```python
from build123d import *

# Parameters (mm, degrees)
F0_W     = 1143
F0_H     = 635
F1_DEPTH = 25.4
F2_W     = 76.2
F2_H     = 76.2
F3_DEPTH = 889


with BuildPart() as f1:
    # F0 (on Top) → F1 (new body, symmetric)
    with BuildSketch(Plane.XY):
        Rectangle(F0_W, F0_H)
    extrude(amount=F1_DEPTH, both=True)

    # F2 (on face) → F3 (join)
    with BuildSketch(Plane.XY.offset(25.4)):
        with Locations((-533.4, 279.4)):
            Rectangle(F2_W, F2_H)
        with Locations((-533.4, -279.4)):
            Rectangle(F2_W, F2_H)
        with Locations((533.4, 279.4)):
            Rectangle(F2_W, F2_H)
        with Locations((533.4, -279.4)):
            Rectangle(F2_W, F2_H)
    extrude(amount=F3_DEPTH)


solid = f1.part
```
The model under review builds one solid part; all positions refer to its coordinate system, in mm. A direction names the side the tool comes from. Round coordinates to 2 decimals unless told otherwise and drop trailing zeros. Write each loop counter-clockwise with the first axis right and the second up, starting at its lowest first coordinate (ties: lowest second). Pieces come first, ordered by that corner, then holes. Notation, with made-up numbers: (53.5, -13.5) - (90.5, -13.5) arc R30 cw to (90.5, 9.5) - close; hole circle Ø3 at (-9.5, 76). An arc over 180 degrees is marked (long way). Answer as CSV lines item,"result". Start each with the question number.
(1) To check wall thickness, follow line 1 (Y direction, x = 512, z = 719); line 2 (Z direction, x = -198, y = -113.5). State the ranges of each line that lie inside material, in increasing order.
(2) For faces 1 (the flat face through (495.3, -280, 464)), 2 (the flat face through (533, -241.3, 464)), 3 (the flat face through (571.5, -260, 377)), list the 3-axis set-ups (+Z, -Z, +X, -X, +Y, -Y) from which the entire face can be reached by the end or side of a thin tool; tool diameter is ignored.
(3) Draft analysis for pull direction X (two halves, no side actions). For faces 4 (the flat face through (-571.5, -260, 338)), 5 (the flat face through (533, 241.3, 464)), 6 (the flat face through (-8, 4, 25.4)), state which applies: pulls with the +X half, pulls with the -X half, needs draft (parallel to the pull), parting line crosses it, or undercut.
(4) We need section A-A on z = 473.5. State the section outline as (x, y) points.
(5) We need section C-C on x = 185. State the section outline as (y, z) points, plus the area to 3 significant figures.
(6) We need section B-B on y = -213.5. State the section outline as (x, z) points, plus the area to 3 significant figures.
Worked answers:
1,line 1,"-317.5 to -241.3, 241.3 to 317.5"
1,line 2,"-25.4 to 25.4"
2,face 1,"+Z, +Y, -Y"
2,face 2,"+Z, +X, -X"
2,face 3,"+Z, -Z, +X, +Y, -Y"
3,face 4,"pulls with the -X half"
3,face 5,"needs draft"
3,face 6,"undercut"
4,outline,"(-571.5, -317.5) - (-495.3, -317.5) - (-495.3, -241.3) - (-571.5, -241.3) - close; (-571.5, 241.3) - (-495.3, 241.3) - (-495.3, 317.5) - (-571.5, 317.5) - close; (495.3, -317.5) - (571.5, -317.5) - (571.5, -241.3) - (495.3, -241.3) - close; (495.3, 241.3) - (571.5, 241.3) - (571.5, 317.5) - (495.3, 317.5) - close"
5,outline,"(-317.5, -25.4) - (317.5, -25.4) - (317.5, 25.4) - (-317.5, 25.4) - close"
5,area,"32,300 mm²"
6,outline,"(-571.5, -25.4) - (571.5, -25.4) - (571.5, 25.4) - (-571.5, 25.4) - close"
6,area,"58,100 mm²"
